from build123d import *

# Parameters (mm, degrees)
SKETCH2_W           = 60
SKETCH2_H           = 13.5
SKETCH2_R           = 1.75
BOSS_EXTRUDE1_DEPTH = 10
BOSS_EXTRUDE2_DEPTH = 21.5
BOSS_EXTRUDE3_DEPTH = 60
SKETCH10_R          = 1.3
CUT_EXTRUDE1_DEPTH  = 22.5
SKETCH12_W          = 14.2
SKETCH12_H          = 32.2
CUT_EXTRUDE2_DEPTH  = 12
CUT_EXTRUDE3_DEPTH  = 12
SKETCH14_R          = 3
CUT_EXTRUDE4_DEPTH  = 6.5
SKETCH15_R          = 1.6
SKETCH15_R_2        = 1.5
SKETCH15_W          = 8.2
SKETCH15_H          = 8.2
CUT_EXTRUDE5_DEPTH  = 22.5
CUT_EXTRUDE6_DEPTH  = 8
BOSS_EXTRUDE4_DEPTH = 60


with BuildPart() as part:
    # Sketch2 → Boss-Extrude1 (new body)
    with BuildSketch(Plane(origin=(0, 0, 0), x_dir=(1, 0, 0), z_dir=(0, 1, 0))):
        with Locations((14.63, 1.75)):
            Rectangle(SKETCH2_W, SKETCH2_H)
        Circle(SKETCH2_R, mode=Mode.SUBTRACT)
        with Locations((29.264, 0)):
            Circle(SKETCH2_R, mode=Mode.SUBTRACT)
    extrude(amount=BOSS_EXTRUDE1_DEPTH)



with BuildPart() as body_2:
    # Sketch5 → Boss-Extrude2 (new body)
    with BuildSketch(Plane(origin=(0, 0, 0), x_dir=(1, 0, 0), z_dir=(0, 1, 0))):
        Polygon((-15.37, 8.5), (-15.37, 33.533725193), (-23.847078232, 33.533725193), (5.995022283, 115.524222507), (23.264977717, 115.524222507), (53.301097121, 33.000662678), (44.63, 33.000662678), (44.63, 8.5), align=None)
    extrude(amount=-BOSS_EXTRUDE2_DEPTH)


with BuildPart() as part_1:
    add(part.part)

    add(body_2.part)  # Boss-Extrude3 merges body 2
    # Sketch8 → Boss-Extrude3 (add)
    with BuildSketch(Plane.ZY.offset(15.37)):
        with BuildLine():
            Line((-18.5, 0), (-8.5, 0))
            Line((-8.5, 0), (-8.5, 10))
            ThreePointArc((-8.5, 10), (-11.428932188, 2.928932188), (-18.5, 0))
        make_face()
    extrude(amount=-BOSS_EXTRUDE3_DEPTH)

    # Sketch10 → Cut-Extrude1 (cut, through all)
    with BuildSketch(Plane(origin=(0, 0, 0), x_dir=(1, 0, 0), z_dir=(0, 1, 0))):
        with Locations((19.38, 112.769736608)):
            Circle(SKETCH10_R)
        with Locations((9.88, 112.769736608)):
            Circle(SKETCH10_R)
    extrude(amount=-CUT_EXTRUDE1_DEPTH, mode=Mode.SUBTRACT)

    # Sketch12 → Cut-Extrude2 (cut)
    with BuildSketch(Plane.XZ.offset(21.5)):
        with Locations((14.63, -93.8)):
            Rectangle(SKETCH12_W, SKETCH12_H)
        with Locations((-4.57, -40.6)):
            Rectangle(SKETCH12_W, SKETCH12_H)
        with Locations((14.63, -40.6)):
            Rectangle(SKETCH12_W, SKETCH12_H)
        with Locations((33.83, -40.6)):
            Rectangle(SKETCH12_W, SKETCH12_H)
    extrude(amount=-CUT_EXTRUDE2_DEPTH, mode=Mode.SUBTRACT)

    # Sketch13 → Cut-Extrude3 (cut)
    with BuildSketch(Plane.XZ.offset(21.5)):
        Polygon((21.73, -77.7), (7.53, -77.7), (7.53, -61.7), (7.53, -57.396998359), (22.223753722, -57.396998359), (22.223753722, -8.5), (21.73, -8.5), (21.73, -24.5), (7.53, -24.5), (7.53, -8.5), (2.53, -8.5), (2.53, -24.5), (-11.67, -24.5), (-11.67, -8.5), (-11.67, -5.014735678), (40.93, -5.014735678), (40.93, -8.5), (40.93, -24.5), (26.73, -24.5), (26.73, -8.5), (26.149155121, -8.5), (26.149155121, -61.7), (21.73, -61.7), align=None)
    extrude(amount=-CUT_EXTRUDE3_DEPTH, mode=Mode.SUBTRACT)

    # Sketch14 → Cut-Extrude4 (cut)
    with BuildSketch(Plane(origin=(0, 10, 0), x_dir=(1, 0, 0), z_dir=(0, 1, 0))):
        Circle(SKETCH14_R)
        with Locations((29.264, 0)):
            Circle(SKETCH14_R)
    extrude(amount=-CUT_EXTRUDE4_DEPTH, mode=Mode.SUBTRACT)

    # Sketch15 → Cut-Extrude5 (cut, through all)
    with BuildSketch(Plane(origin=(0, 0, 0), x_dir=(1, 0, 0), z_dir=(0, 1, 0))):
        with Locations((-4.57, 31.6)):
            Circle(SKETCH15_R)
        with Locations((14.63, 31.6)):
            Circle(SKETCH15_R)
        with Locations((33.83, 31.6)):
            Circle(SKETCH15_R_2)
        with Locations((14.63, 84.8)):
            Circle(SKETCH15_R)
        with Locations((17.63, 93.8)):
            Rectangle(SKETCH15_W, SKETCH15_H)
        with Locations((17.63, 39.4)):
            Rectangle(SKETCH15_W, SKETCH15_H)
        with Locations((36.83, 39.4)):
            Rectangle(SKETCH15_W, SKETCH15_H)
        with Locations((-1.57, 39.4)):
            Rectangle(SKETCH15_W, SKETCH15_H)
    extrude(amount=-CUT_EXTRUDE5_DEPTH, mode=Mode.SUBTRACT)

    # Sketch16 → Cut-Extrude6 (cut)
    with BuildSketch(Plane(origin=(0, 0, 0), x_dir=(1, 0, 0), z_dir=(0, 1, 0))):
        Polygon((-15.37, 18.5), (44.63, 18.5), (44.63, 33.000662678), (53.301097121, 33.000662678), (23.264977717, 115.524222507), (5.995022283, 115.524222507), (-23.847078232, 33.533725193), (-15.37, 33.533725193), align=None)
    extrude(amount=-CUT_EXTRUDE6_DEPTH, mode=Mode.SUBTRACT)

    # Sketch17 → Boss-Extrude4 (add)
    with BuildSketch(Plane(origin=(44.63, 0, 0), x_dir=(0, 0, -1), z_dir=(1, 0, 0))):
        Polygon((18.5, 0), (25.750331339, -8), (18.5, -8), align=None)
    extrude(amount=-BOSS_EXTRUDE4_DEPTH)


solid = part_1.part
Build history of the part. All positions in model axes, mm. A direction names the side the tool comes from. Round coordinates to 2 decimals unless told otherwise and drop trailing zeros. Write each loop counter-clockwise with the first axis right and the second up, starting at its lowest first coordinate (ties: lowest second). Pieces come first, ordered by that corner, then holes. Notation, with made-up numbers: M 53,-23.75 L 90,-23.75 A12 cw 90,-1.75 Z; hole C -40,55.5 d4. An arc over 180 degrees is marked long. Answer as a JSON object with one key per item and string values. Group by question number.
(1) Cut at D-D (x = 19.38). Give the cut face in (y, z), and give its area (3 significant figures).
(2) Cut at A-A (z = -31.6). Give the number of separate pieces and of enclosed holes in the cut face, and give its area (3 significant figures).
(3) Flat gauge pins, fed straight in: pin 1 (1 mm diameter, centred on y = -11, z = -16, fed in from +X); pin 2 (2.5 mm diameter, centred on x = -19.5, y = -11.5, fed in from +Z); pin 3 (12 mm diameter, centred on y = -7.5, z = -79.5, fed in from +X); pin 4 (4 mm diameter, centred on x = -8.5, z = -83, fed in from +Y). Where does each tip first touch, or does it go through?
(4) Mould opens along X. For faces 5 (the flat face through (14, 0, -2)), 6 (the cylindrical face through (30.93, 1.73, -0.53)), 7 (the flat face through (44.63, -9, -14)) say: pulls with the +X half, pulls with the -X half, needs draft (parallel to the pull), parting line crosses it, or undercut.
(5) Cut at B-B (x = 9.88). Give the cut face in (y, z).
(6) Drill centre lines: L1, parallel to X at y = -8.65, z = -31.6; L2, parallel to X at y = -18.5, z = -23.5; L3, parallel to Z at x = 19.38, y = -18.25. Where is each one in solid material? Low to high.
(7) Which spindle directions (+Z, -Z, +X, -X, +Y, -Y) get a long thin tool onto all of the face, cutting with end or side? Do faces 1 (the flat face through (-15.37, -9, -15)), 2 (the cylindrical face through (32.125, 6.796, -0.901)), 3 (the flat face through (15, -6, -8.5)), 4 (the flat face through (7.53, -16, -83)). Say none if no direction does.
(8) Cut at C-C (z = 0). Give the cut face in (x, y), and give its area (4 significant figures).
Responses:
{
 "1": {"outline": "M -21.5,-115.52 L -8,-115.52 L -8,-114.07 L -21.5,-114.07 Z; M -21.5,-111.47 L -8,-111.47 L -8,-97.9 L -9.5,-97.9 L -9.5,-109.9 L -21.5,-109.9 Z; M -21.5,-57.4 L -9.5,-57.4 L -9.5,-89.7 L -8,-89.7 L -8,-43.5 L -9.5,-43.5 L -9.5,-56.7 L -21.5,-56.7 Z; M -9.5,-35.3 L -8,-35.3 L -8,-25.75 L 0,-18.5 A10 cw 10,-8.5 L 10,5 L 0,5 L 0,-8.5 L -9.5,-8.5 Z", "area": "442 mm2"},
 "2": {"separate pieces": "4", "enclosed holes": "0", "area": "238 mm2"},
 "3": {"pin 1": "stops at x = 44.63", "pin 2": "stops at z = -33.53", "pin 3": "stops at x = 38.55", "pin 4": "passes through"},
 "4": {"face 5": "needs draft", "face 6": "undercut", "face 7": "pulls with the +X half"},
 "5": {"outline": "M -21.5,-115.52 L -8,-115.52 L -8,-114.07 L -21.5,-114.07 Z; M -21.5,-111.47 L -8,-111.47 L -8,-25.75 L 0,-18.5 A10 cw 10,-8.5 L 10,5 L 0,5 L 0,-8.5 L -9.5,-8.5 L -9.5,-56.7 L -21.5,-56.7 L -21.5,-57.4 L -9.5,-57.4 L -9.5,-109.9 L -21.5,-109.9 Z"},
 "6": {"L1": "x = -15.37 to -6.17, -2.97 to 13.03, 16.23 to 32.33, 35.33 to 44.63", "L2": "x = -15.37 to -11.67, 2.53 to 7.53, 21.73 to 22.22, 26.15 to 26.73, 40.93 to 44.63", "L3": "z = -115.52 to -114.07, -111.47 to -109.9, -57.4 to -56.7"},
 "7": {"face 1": "+Z, -X, +Y, -Y", "face 2": "+Y", "face 3": "+Z, +X, -X, -Y", "face 4": "-Y"},
 "8": {"outline": "M -15.37,0 L -1.75,0 L -1.75,3.5 L -3,3.5 L -3,10 L -15.37,10 Z; M 1.75,0 L 27.51,0 L 27.51,3.5 L 26.26,3.5 L 26.26,10 L 3,10 L 3,3.5 L 1.75,3.5 Z; M 31.01,0 L 44.63,0 L 44.63,10 L 32.26,10 L 32.26,3.5 L 31.01,3.5 Z", "area": "497.5 mm2"}
}
